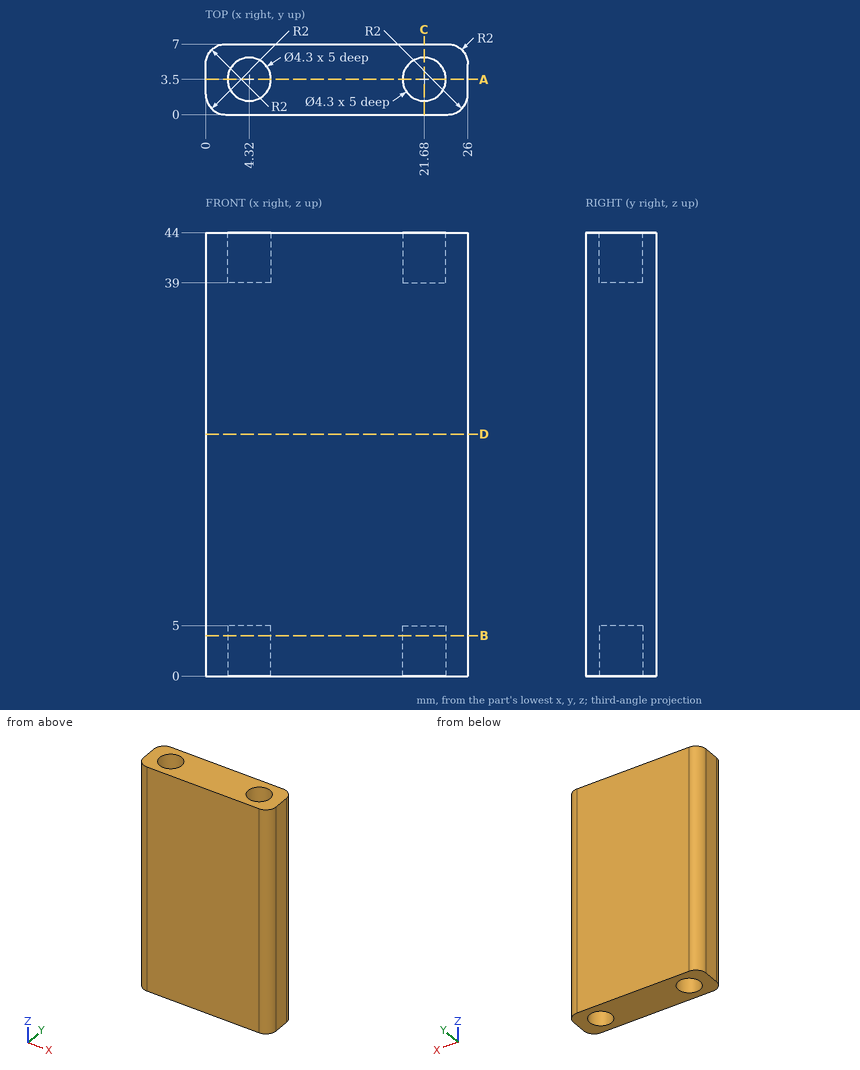
Study the drawing (mm; zero at the part's minimum x, y, z) and answer. Round coordinates to 2 decimals unless told otherwise and drop trailing zeros. Loops run counter-clockwise (first coordinate to the right, second up) from the corner with the lowest first, then second, coordinate; pieces in that order, holes last. Notation, with made-up numbers: (35, 12.5) -> (86, 12.5) arc R23 cw to (86, 29.5) -> close; hole circle Ø10 at (31, 75.5). An arc over 180 degrees is marked (long way). One line per item, written item: value.
1) Flat-ended cylindrical pins translate along their axes: P1, Ø3.5, axis at x = 3.5, y = 3, coming from the +Z side; P2, Ø4, axis at x = 4.32, y = 3.5, coming from the +Z side. Find the tip coordinate at first contact, or state that the pin passes through.
Answer list:
P1: stops at z = 44
P2: stops at z = 39
2) A cutting plane is placed at C-C (x = 21.68). Determine the outline of the cut face in (y, z), and give its area (3 significant figures).
Answer list:
outline: (0, 0) -> (1.35, 0) -> (1.35, 5) -> (5.65, 5) -> (5.65, 0) -> (7, 0) -> (7, 44) -> (5.65, 44) -> (5.65, 39) -> (1.35, 39) -> (1.35, 44) -> (0, 44) -> close
area: 265 mm²
3) A cutting plane is placed at D-D (z = 24). Determine the outline of the cut face in (x, y).
Answer list:
outline: (0, 2) arc R2 ccw to (2, 0) -> (24, 0) arc R2 ccw to (26, 2) -> (26, 5) arc R2 ccw to (24, 7) -> (2, 7) arc R2 ccw to (0, 5) -> close
4) A cutting plane is placed at A-A (y = 3.5). Determine the outline of the cut face in (x, z), and give its area (3 significant figures).
Answer list:
outline: (0, 0) -> (2.17, 0) -> (2.17, 5) -> (6.47, 5) -> (6.47, 0) -> (19.53, 0) -> (19.53, 5) -> (23.83, 5) -> (23.83, 0) -> (26, 0) -> (26, 44) -> (23.83, 44) -> (23.83, 39) -> (19.53, 39) -> (19.53, 44) -> (6.47, 44) -> (6.47, 39) -> (2.17, 39) -> (2.17, 44) -> (0, 44) -> close
area: 1,060 mm²
5) A cutting plane is placed at B-B (z = 4). Determine the outline of the cut face in (x, y).
Answer list:
outline: (0, 2) arc R2 ccw to (2, 0) -> (24, 0) arc R2 ccw to (26, 2) -> (26, 5) arc R2 ccw to (24, 7) -> (2, 7) arc R2 ccw to (0, 5) -> close; hole circle Ø4.3 at (4.32, 3.5); hole circle Ø4.3 at (21.68, 3.5)
6) Consider L1, parallel to Y at x = 4.32, z = 1.6; L2, parallel to Z at x = 2.75, y = 4.25; L3, parallel to X at y = 1.5, z = 26.5. Determine where each line is inside the solid, lowest interval first. Write a range as [from, to].
Answer list:
L1: y = [0, 1.35], [5.65, 7]
L2: z = [5, 39]
L3: x = [0.06, 25.94]
